For this review, use the dimensioned drawing (mm, ordinates from the lowest corner) and the shaded views. A direction names the side the tool comes from. Coordinates: 2 decimals unless noted, no trailing zeros. Loops run counter-clockwise (first coordinate to the right, second up) from the corner with the lowest first, then second, coordinate; pieces in that order, holes last. Notation, with made-up numbers: (33.25, -34.5) - (68.25, -34.5) arc R17 cw to (68.25, -6.5) - close; hole circle Ø3 at (86.25, -5). An arc over 180 degrees is marked (long way). Answer in a Markdown table with one row per item. Add a question column.
(1) We need section A-A, the plane z = 6. Write out the cut boundary in (x, y).
(2) We need section D-D, the plane x = 141. Write out the cut boundary in (y, z).
(3) We need section B-B, the plane x = 51. Write out the cut boundary in (y, z), plus the area to 3 significant figures.
(4) Clearance check with flat-ended pins moving along their axes: pin 1 (6 mm diameter, centred on y = 100, z = 9, fed in from -X); pin 2 (3 mm diameter, centred on y = 150.5, z = 6.5, fed in from +X); pin 3 (1 mm diameter, centred on x = 51.5, z = 13, fed in from -Y). State where each tip first meets the part, or that it passes through.
(5) We need section C-C, the plane y = 75. Write out the cut boundary in (x, z), plus the area to 3 significant figures.
(6) To check wall thickness, follow L1, parallel to Y at x = 180.5, z = 3.5; L2, parallel to X at y = 84, z = 5; L3, parallel to Z at x = 153, y = 159. State the ranges of each line that lie inside material, in increasing order. Write a range as [from, to].
(7) For the marked faces 1, 2 and 3, list the 3-axis set-ups (+Z, -Z, +X, -X, +Y, -Y) from which the entire face can be reached by the end or side of a thin tool; tool diameter is ignored.
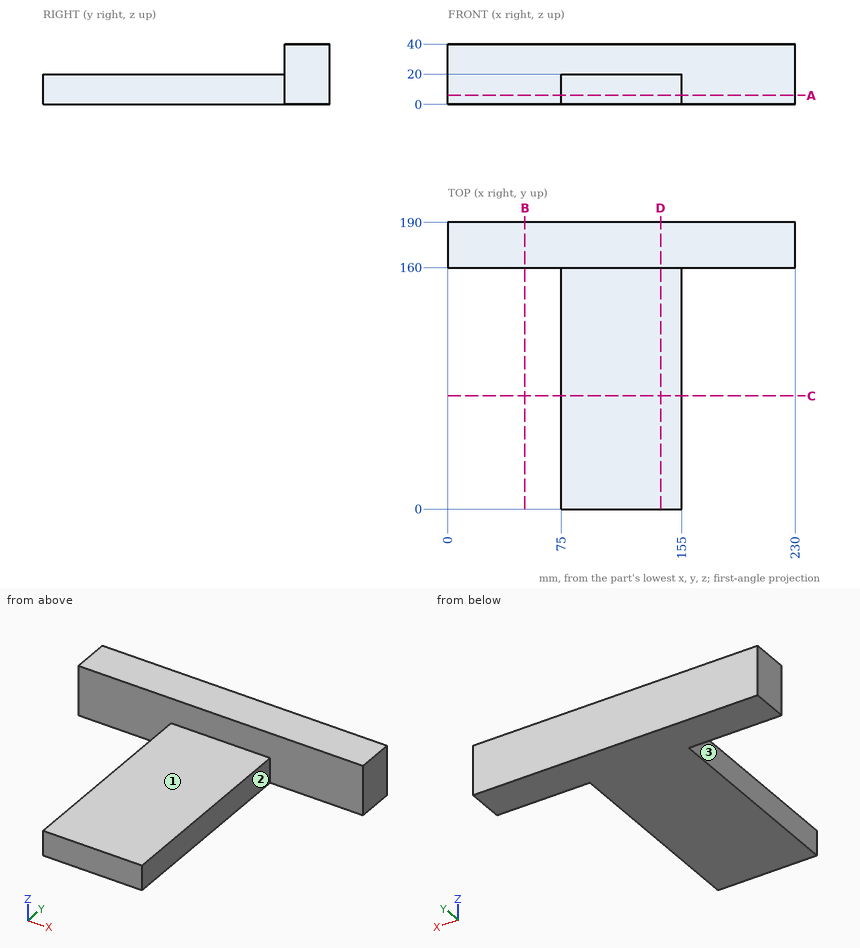
Responses:
| question | item | result |
|---|---|---|
| 1 | outline | (0, 160) - (75, 160) - (75, 0) - (155, 0) - (155, 160) - (230, 160) - (230, 190) - (0, 190) - close |
| 2 | outline | (0, 0) - (190, 0) - (190, 40) - (160, 40) - (160, 20) - (0, 20) - close |
| 3 | outline | (160, 0) - (190, 0) - (190, 40) - (160, 40) - close |
| 3 | area | 1,200 mm2 |
| 4 | pin 1 | stops at x = 75 |
| 4 | pin 2 | stops at x = 155 |
| 4 | pin 3 | stops at y = 160 |
| 5 | outline | (75, 0) - (155, 0) - (155, 20) - (75, 20) - close |
| 5 | area | 1,600 mm2 |
| 6 | L1 | y = [160, 190] |
| 6 | L2 | x = [75, 155] |
| 6 | L3 | z = [0, 20] |
| 7 | face 1 | +Z, +X, -X, -Y |
| 7 | face 2 | +Z, -Z, +X, -Y |
| 7 | face 3 | +Z, -Z, -X, -Y |
